Model file for the job. Use its own axes, mm. Face numbers are marked on the shaded views. A direction names the side the tool comes from. Round coordinates to 2 decimals unless told otherwise and drop trailing zeros. Order: outer loops, then holes, each group sorted by start corner. A loop starts at its lowest first (then second) coordinate and runs counter-clockwise, first axis right, second up. Notation, with made-up numbers: (78, -23.5) -> (131, -23.5) arc R18 ccw to (131, -7.5) -> close; hole circle Ø5 at (74, 38). An arc over 180 degrees is marked (long way). Answer as CSV lines item,"result".
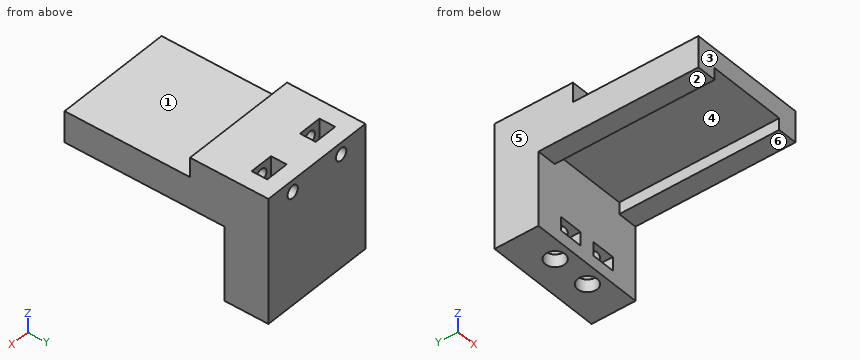
```python
from build123d import *

# Parameters (mm, degrees)
SKETCH_2_W          = 30
SKETCH_2_H          = 52
EXTRUDE_1_DEPTH     = 5
SKETCH_3_W          = 5
SKETCH_3_H          = 40.81
EXTRUDE_2_DEPTH     = 3
SKETCH_4_W          = 30
SKETCH_4_H          = 10
EXTRUDE_3_DEPTH     = 20
SKETCH_6_R          = 1.6
CUT_EXTRUDE_1_DEPTH = 15
SKETCH_7_W          = 6
SKETCH_7_H          = 4
CUT_EXTRUDE_2_DEPTH = 6
SKETCH_8_W          = 30
SKETCH_8_H          = 11.19
EXTRUDE_4_DEPTH     = 22
SKETCH_9_R          = 2.5
CUT_EXTRUDE_3_DEPTH = 10
SKETCH_10_W         = 6
SKETCH_10_H         = 3.5
CUT_EXTRUDE_4_DEPTH = 8


with BuildPart() as part:
    # 草图2 → 凸台-拉伸1 (new body)
    with BuildSketch(Plane.XY):
        with Locations((0, -11.302890995)):
            Rectangle(SKETCH_2_W, SKETCH_2_H)
    extrude(amount=EXTRUDE_1_DEPTH)

    # 草图3 → 凸台-拉伸2 (add)
    with BuildSketch(Plane.XY):
        with Locations((-12.5, -16.897890995)):
            Rectangle(SKETCH_3_W, SKETCH_3_H)
        with Locations((12.5, -16.897890995)):
            Rectangle(SKETCH_3_W, SKETCH_3_H)
    extrude(amount=-EXTRUDE_2_DEPTH)

    # 草图4 → 凸台-拉伸3 (add)
    with BuildSketch(Plane(origin=(0, 14.697109005, 0), x_dir=(1, 0, 0), z_dir=(0, 1, 0))):
        with Locations((0, -5)):
            Rectangle(SKETCH_4_W, SKETCH_4_H)
    extrude(amount=-EXTRUDE_3_DEPTH)

    # 草图6 → 切除-拉伸1 (cut)
    with BuildSketch(Plane(origin=(0, 14.697109005, 0), x_dir=(1, 0, 0), z_dir=(0, 1, 0))):
        with Locations((-7.5, -7)):
            Circle(SKETCH_6_R)
        with Locations((7.5, -7)):
            Circle(SKETCH_6_R)
    extrude(amount=-CUT_EXTRUDE_1_DEPTH, mode=Mode.SUBTRACT)

    # 草图7 → 切除-拉伸2 (cut)
    with BuildSketch(Plane.XY.offset(10)):
        with Locations((-7.5, 8.697109005)):
            Rectangle(SKETCH_7_W, SKETCH_7_H)
        with Locations((7.5, 8.697109005)):
            Rectangle(SKETCH_7_W, SKETCH_7_H)
    extrude(amount=-CUT_EXTRUDE_2_DEPTH, mode=Mode.SUBTRACT)

    # 草图8 → 凸台-拉伸4 (add)
    with BuildSketch(Plane.XY):
        with Locations((0, 9.102109005)):
            Rectangle(SKETCH_8_W, SKETCH_8_H)
    extrude(amount=-EXTRUDE_4_DEPTH)

    # 草图9 → 切除-拉伸3 (cut)
    with BuildSketch(Plane(origin=(0, 0, -22), x_dir=(-1, 0, 0), z_dir=(0, 0, -1))):
        with Locations((-5, 7.507109005)):
            Circle(SKETCH_9_R)
        with Locations((5, 7.507109005)):
            Circle(SKETCH_9_R)
    extrude(amount=-CUT_EXTRUDE_3_DEPTH, mode=Mode.SUBTRACT)

    # 草图10 → 切除-拉伸4 (cut)
    with BuildSketch(Plane(origin=(0, 3.507109005, 0), x_dir=(-1, 0, 0), z_dir=(0, -1, 0))):
        with Locations((5, 17)):
            Rectangle(SKETCH_10_W, SKETCH_10_H)
        with Locations((-5, 17)):
            Rectangle(SKETCH_10_W, SKETCH_10_H)
    extrude(amount=-CUT_EXTRUDE_4_DEPTH, mode=Mode.SUBTRACT)


solid = part.part
```
Q1. Flat gauge pins, fed straight in: pin 1 (1.8 mm diameter, centred on x = -4.5, y = 6.5, fed in from -Z); pin 2 (12 mm diameter, centred on x = -1.5, z = -12, fed in from -Y); pin 3 (4 mm diameter, centred on x = 4.5, y = -19.5, fed in from +Z). Where does each tip first touch, or does it go through?
Checks:
pin 1,"z = -12"
pin 2,"y = 3.51"
pin 3,"z = 5"
Q2. Wall check: L1, parallel to X at y = 13, z = 7; L2, parallel to Y at x = 5, z = -12.7; L3, parallel to Z at x = -7.5, y = 3. Give the ranges that are in metal, low to high. Write a range as [from, to].
Checks:
L1,"[-15, -9.1], [-5.9, 5.9], [9.1, 15]"
L2,"[3.51, 5.01], [10.01, 14.7]"
L3,"[0, 5.4], [8.6, 10]"
Q3. Tool access for the marked faces 1, 2 and 3: list every direction of +Z, -Z, +X, -X, +Y, -Y with a clear straight run to the whole face (end or side of a thin tool).
Checks:
face 1,"+Z, +X, -X, -Y"
face 2,"-Z, +X, -X, -Y"
face 3,"+Z, -Z, +X, -X, -Y"
Q4. Mould opens along X. For the marked faces 4, 5 and 6 say: +X half, -X half, draft (parallel to the pull), parting line (faces both ways), or undercut.
Checks:
face 4,"undercut"
face 5,"-X half"
face 6,"draft"
Q5. Saw through at C-C (y = -29). Write the cut outline in (x, z), plus the area to 3 significant figures.
Checks:
outline,"(-15, -3) -> (-10, -3) -> (-10, 0) -> (10, 0) -> (10, -3) -> (15, -3) -> (15, 5) -> (-15, 5) -> close"
area,"180 mm²"
Q6. Saw through at A-A (z = -17). Write the cut outline in (x, y).
Checks:
outline,"(-15, 3.51) -> (-8, 3.51) -> (-8, 11.51) -> (-2, 11.51) -> (-2, 3.51) -> (2, 3.51) -> (2, 11.51) -> (8, 11.51) -> (8, 3.51) -> (15, 3.51) -> (15, 14.7) -> (-15, 14.7) -> close"
Q7. Saw through at B-B (x = 12.5). Write the cut outline in (y, z).
Checks:
outline,"(-37.3, -3) -> (3.51, -3) -> (3.51, -22) -> (14.7, -22) -> (14.7, 10) -> (-5.3, 10) -> (-5.3, 5) -> (-37.3, 5) -> close"
Q8. Saw through at D-D (z = -13). Write the cut outline in (x, y), plus the area to 3 significant figures.
Checks:
outline,"(-15, 3.51) -> (15, 3.51) -> (15, 14.7) -> (-15, 14.7) -> close; hole circle Ø5 at (-5, 7.51); hole circle Ø5 at (5, 7.51)"
area,"296 mm²"
